Read the model definition and answer for the solid it produces. Units are mm, in the model's axes. A direction names the side the tool comes from. Give positions to 0.01 mm unless a question says otherwise; leave off trailing zeros. Write each loop counter-clockwise with the first axis right and the second up, starting at its lowest first coordinate (ties: lowest second). Pieces come first, ordered by that corner, then holes. Notation, with made-up numbers: M 9.25,23.25 L 59.25,23.25 A5 ccw 59.25,31.25 Z; hole C 68.5,60.25 d11. An arc over 180 degrees is marked long. Put each result on its own line as item: value.
Autodesk Inventor part; units mm, degrees
ref_plane "YZ Plane" through (0, 0, 0) normal (1, 0, 0) x (0, 1, 0)
ref_plane "XZ Plane" through (0, 0, 0) normal (0, 1, 0) x (-1, 0, 0)
ref_plane "XY Plane" through (0, 0, 0) normal (0, 0, 1) x (1, 0, 0)
sketch "Sketch1" plane through (0, 0, 0) normal (0, 1, 0) x (-1, 0, 0)
  line L0 (4.385, 55) -> (0.885, 55)
  line L1 (0.885, 55) -> (0.885, 5)
  line L2 (0.885, 5) -> (4.385, 5)
  line L3 (4.385, 5) -> (4.385, 55)
  line L4 (-0.865, 5) -> (-4.365, 5)
  line L5 (-4.365, 5) -> (-4.365, 55)
  line L6 (-4.365, 55) -> (-0.865, 55)
  line L7 (-0.865, 55) -> (-0.865, 5)
  line L8 (0.885, 5) -> (-0.865, 5)
  line L9 (-0.865, 55) -> (0.885, 55)
  line L10 (4.365, -5) -> (0.865, -5)
  line L11 (0.865, -5) -> (0.865, -55)
  line L12 (0.865, -55) -> (4.365, -55)
  line L13 (4.365, -55) -> (4.365, -5)
  line L14 (-0.885, -55) -> (-4.385, -55)
  line L15 (-4.385, -55) -> (-4.385, -5)
  line L16 (-4.385, -5) -> (-0.885, -5)
  line L17 (-0.885, -5) -> (-0.885, -55)
  line L18 (-0.885, -5) -> (0.865, -5)
  line L19 (0.865, -55) -> (-0.885, -55)
  line L20 (55, -4.375) -> (15, -4.375)
  line L21 (15, -4.375) -> (15, -0.875)
  line L22 (15, -0.875) -> (55, -0.875)
  line L23 (55, -0.875) -> (55, -4.375)
  line L24 (15, 0.875) -> (55, 0.875)
  line L25 (55, 0.875) -> (55, 4.375)
  line L26 (55, 4.375) -> (15, 4.375)
  line L27 (15, 4.375) -> (15, 0.875)
  line L28 (-15, -4.375) -> (-55, -4.375)
  line L29 (-55, -4.375) -> (-55, -0.875)
  line L30 (-55, -0.875) -> (-15, -0.875)
  line L31 (-15, -0.875) -> (-15, -4.375)
  line L32 (-55, 0.875) -> (-15, 0.875)
  line L33 (-15, 0.875) -> (-15, 4.375)
  line L34 (-15, 4.375) -> (-55, 4.375)
  line L35 (-55, 4.375) -> (-55, 0.875)
  line L36 (-15, 0.875) -> (-15, -0.875) construction
  line L37 (-55, -0.875) -> (-55, 0.875) construction
  line L38 (15, 0.875) -> (15, -0.875) construction
  line L39 (55, -0.875) -> (55, 0.875) construction
  line L40 (15, -4.375) -> (-15, -4.375) construction
  line L41 (-15, 4.375) -> (15, 4.375) construction
  line L42 (15, -4.375) -> (0, 0) construction
  line L43 (0, 0) -> (-15, -4.375) construction
  line L44 (-15, 4.375) -> (0, 0) construction
  line L45 (-4.385, -5) -> (0, 0) construction
  line L46 (0, 0) -> (4.385, 5) construction
  line L47 (0, 0) -> (4.365, -5) construction
  line L48 (0, 0) -> (-4.365, 5) construction
  point P0 (-0.01, -5)
  point P1 (0.01, 5)
  dimension "d0" = 1.75
  dimension "d2" = 110
  dimension "d3" = 3.5
  dimension "d5" = 40
  dimension "d15" = 30
  dimension "d16" = 10
  dimension "d21" = 0.01
extrude "Extrusion1" add sketch "Sketch1" along normal blind 6.35 contours L20 L21 L22 L23 | L27 L26 L25 L24 | L28 L29 L30 L31 | L35 L34 L33 L32
extrude "Extrusion3" add sketch "Sketch1" along normal blind 17.25 contours L3 L2 L1 L0 | L7 L4 L5 L6 | L13 L12 L11 L10 | L17 L14 L15 L16
sketch "Sketch2" plane through (0, 0, 0) normal (0, -1, 0) x (1, 0, 0)
  circle A0 centre (0, 0) radius 62.23
  dimension "d8" = 124.46
extrude "Extrusion2" add sketch "Sketch2" along normal blind 3
extrude "Extrusion4" add sketch "Sketch1" along normal blind 14.8 contours L3 L2 L1 L0 | L1 L8 L7 L9 | L7 L4 L5 L6 | L13 L12 L11 L10 | L11 L19 L17 L18 | L17 L14 L15 L16
properties part number "Soldering Jig"
(1) Section A-A on y = 11.25 is taken. Determine the outline of the cut face in (x, z) (3 decimals), and give its area (3 significant figures).
Result:
outline: M -4.385,5 L 4.365,5 L 4.365,55 L -4.385,55 Z; M -4.365,-55 L 4.385,-55 L 4.385,-5 L -4.365,-5 Z
area: 875 mm²
(2) For a pull along Z with two mould halves and no side action, classify faces 5 (the face through (-3, 17.25, -30)), 6 (the face through (0, 9, -5)), 7 (the face through (-13.49, -1.48, 60.75)), 8 (the face through (35, 3, -0.875)) as +Z half, -Z half, draft (parallel to the pull), parting line (faces both ways), or undercut.
Result:
face 5: draft
face 6: undercut
face 7: parting line
face 8: undercut
(3) Section B-B on z = 13 is taken. Determine the outline of the cut face in (x, y) (3 decimals), and give its area (3 significant figures).
Result:
outline: M -60.857,-3 L 60.857,-3 L 60.857,0 L 4.365,0 L 4.365,17.25 L 0.865,17.25 L 0.865,14.8 L -0.885,14.8 L -0.885,17.25 L -4.385,17.25 L -4.385,0 L -60.857,0 Z
area: 512 mm²
(4) Section C-C on x = -48 is taken. Determine the outline of the cut face in (y, z) (3 decimals), and give its area (3 significant figures).
Result:
outline: M -3,-39.605 L 0,-39.605 L 0,-4.375 L 6.35,-4.375 L 6.35,-0.875 L 0,-0.875 L 0,0.875 L 6.35,0.875 L 6.35,4.375 L 0,4.375 L 0,39.605 L -3,39.605 Z
area: 282 mm²
(5) Which of the six approach directions +Z, -Z, +X, -X, +Y, -Y give full straight-line access (tool end or side, diameter ignored) to faces 1 (the face through (-35, 3, 0.875)), 2 (the face through (4.385, 9, -30)), 3 (the face through (0, 9, -55)), 4 (the face through (-15, 3, 3))?
Result:
face 1: +X, -X, +Y
face 2: +Z, -Z, +X, +Y
face 3: -Z, +X, -X, +Y
face 4: +Z, -Z, +Y
(6) Given pin 1 Ø1.5 at (x, y) = (32, 3.5) entering from -Z (3 decimals); pin 2 Ø3 at (x, z) = (44.5, 2) entering from +Y; pin 3 Ø3 at (x, y) = (33.5, 3.5) entering from +Z (3 decimals); pin 4 Ø8 at (x, y) = (-18, 13) entering from +Z, each flat-ended and moving along its own axis, determine where each tip first touches the part or whether it passes through.
Result:
pin 1: stops at z = -4.375
pin 2: stops at y = 6.35
pin 3: stops at z = 4.375
pin 4: passes through
(7) Section D-D on x = -9 is taken. Determine the outline of the cut face in (y, z), and give its area (3 significant figures).
Result:
outline: M -3,-61.58 L 0,-61.58 L 0,61.58 L -3,61.58 Z
area: 369 mm²
(8) Straight lines are drawn through the part: line 1 along X through (y, z) = (11.5, 14) (3 decimals); line 2 along X through (y, z) = (15, -27) (3 decimals); line 3 along Y through (x, z) = (-31.5, 11.5). For each, find the intervals that lie inside material, in ascending order. Write a range as from..to.
Result:
line 1: x = -4.385..4.365
line 2: x = -4.365..-0.865, 0.885..4.385
line 3: y = -3..0
